The model under review builds one solid part; all positions refer to its coordinate system, in mm. A direction names the side the tool comes from. Give positions to 0.01 mm unless a question says otherwise; leave off trailing zeros. Order: outer loops, then holes, each group sorted by start corner. A loop starts at its lowest first (then second) coordinate and runs counter-clockwise, first axis right, second up.
```python
from build123d import *

# Parameters (mm, degrees)
F5_W      = 0.8128
F5_H      = 13.4112
F6_DEPTH  = 25.1968
F8_DEPTH  = 46.8002
F5_W_2    = 19.5072
F5_H_2    = 1.2
F5_W_3    = 5.1816
F5_H_3    = 11.592
F5_W_4    = 17.9008
F5_H_4    = 7.5376
F5_W_5    = 19.1008
F5_H_5    = 4.896
F5_W_6    = 1.2
F5_H_6    = 6.004279983
F9_DEPTH  = 19.4056
F5_W_7    = 4.6104
F5_H_7    = 5.8928
F5_W_8    = 6.1152
F5_H_8    = 4.712
F5_W_9    = 12.8016
F5_W_10   = 8.3888
F5_H_9    = 7.0104
F10_DEPTH = 17.9832
F11_DEPTH = 1.2192
F12_W     = 52.832
F12_H     = 38.2016
F12_W_2   = 1.0041694948
F12_H_2   = 6.004279983
F12_W_3   = 19.1008
F12_H_3   = 16.2133753487
F13_DEPTH = 0.913


with BuildPart() as f6:
    # F5 (on Top) → F6 (new body)
    with BuildSketch(Plane.XY):
        Polygon((0, 36.3344), (0, 0), (46.7992, 0), (46.7992, 1.2), (46.7992, 6.1976), (46.7992, 7.3976), (46.7992, 22.4344), (45.5992, 22.4344), (45.5992, 1.2), (1.2, 1.2), (1.2, 11.36), (1.2, 24.7712), (1.2, 35.1344), (45.5992, 35.1344), (45.5992, 31.864), (46.7992, 31.864), (46.7992, 36.3344), (15.2016, 36.3344), (14.0016, 36.3344), (1.2, 36.3344), align=None)
        with Locations((1.6064, 18.0656)):
            Rectangle(F5_W, F5_H)
    extrude(amount=F6_DEPTH)

    # F7 (on face) → F8 (cut, through all)
    with BuildSketch(Plane(origin=(0, 0, 0), x_dir=(0, -1, 0), z_dir=(-1, 0, 0))):
        Polygon((-35.1344, 25.1968), (0, 19.4056), (0, 25.1968), align=None)
    extrude(amount=-F8_DEPTH, mode=Mode.SUBTRACT)

    # F5 (on Top) → F9 (join)
    with BuildSketch(Plane.XY):
        Polygon((0, 103.7584), (0, 64.3568), (1.2, 64.3568), (1.2, 102.5584), (18.0656, 102.5584), (18.0656, 103.7584), align=None)
        with Locations((27.8192, 103.1584)):
            Rectangle(F5_W_2, F5_H_2)
        Polygon((120.5032, 103.7584), (37.5728, 103.7584), (37.5728, 102.5584), (54.032, 102.5584), (54.032, 64.3568), (55.232, 64.3568), (55.232, 102.5584), (99.0024, 102.5584), (99.0024, 93.8704553318), (100.2024, 93.8704553318), (101.2065694948, 93.8704553318), (101.2065694948, 87.8661753487), (100.2024, 87.8661753487), (99.0024, 87.8661753487), (99.0024, 70.4528), (100.2024, 70.4528), (100.2024, 86.6661753487), (102.4065694948, 86.6661753487), (119.3032, 86.6661753487), (119.3032, 70.4528), (120.5032, 70.4528), align=None)
        Polygon((100.2024, 95.0704553318), (100.2024, 102.5584), (119.3032, 102.5584), (119.3032, 87.8661753487), (102.4065694948, 87.8661753487), (102.4065694948, 95.0704553318), align=None, mode=Mode.SUBTRACT)
        Polygon((46.7992, 7.3976), (46.7992, 6.1976), (59.3152, 6.1976), (59.3152, -3.9624), (59.3152, -5.1624), (60.5152, -5.1624), (119.3032, -5.1624), (120.5032, -5.1624), (120.5032, 70.4528), (119.3032, 70.4528), (100.2024, 70.4528), (99.0024, 70.4528), (99.0024, 64.3568), (55.232, 64.3568), (54.032, 64.3568), (54.032, 63.1568), (66.6304, 63.1568), (66.6304, 36.3344), (67.8304, 36.3344), (67.8304, 63.1568), (119.3032, 63.1568), (119.3032, 49.5424), (100.2024, 49.5424), (100.2024, 36.3344), (101.4024, 36.3344), (101.4024, 39.6048), (119.3032, 39.6048), (119.3032, 21.6216), (107.2128, 21.6216), (107.2128, 20.4216), (119.3032, 20.4216), (119.3032, -3.9624), (92.4808, -3.9624), (92.4808, 20.4216), (91.2808, 20.4216), (91.2808, 8.8296), (86.0992, 8.8296), (86.0992, 20.4216), (84.8992, 20.4216), (84.8992, -3.9624), (60.5152, -3.9624), (60.5152, 20.4216), (59.3152, 20.4216), (59.3152, 7.3976), align=None)
        with Locations((88.69, 1.8336)):
            Rectangle(F5_W_3, F5_H_3, mode=Mode.SUBTRACT)
        with Locations((110.3528, 44.5736)):
            Rectangle(F5_W_4, F5_H_4, mode=Mode.SUBTRACT)
        with Locations((109.7528, 66.8048)):
            Rectangle(F5_W_5, F5_H_5, mode=Mode.SUBTRACT)
        with Locations((99.6024, 90.8683153403)):
            Rectangle(F5_W_6, F5_H_6)
    extrude(amount=F9_DEPTH)

    # F5 (on Top) → F10 (join)
    with BuildSketch(Plane.XY):
        Polygon((0, 64.3568), (0, 36.3344), (1.2, 36.3344), (1.2, 63.1568), (34.5248, 63.1568), (34.5248, 64.3568), (1.2, 64.3568), align=None)
        Polygon((59.3152, 21.6216), (59.3152, 20.4216), (60.5152, 20.4216), (84.8992, 20.4216), (86.0992, 20.4216), (91.2808, 20.4216), (92.4808, 20.4216), (107.2128, 20.4216), (107.2128, 21.6216), (107.2128, 28.7144), (101.4024, 28.7144), (101.4024, 36.3344), (100.2024, 36.3344), (67.8304, 36.3344), (66.6304, 36.3344), (59.3152, 36.3344), (59.3152, 29.2224), (91.4208, 29.2224), (91.4208, 35.1344), (100.2024, 35.1344), (100.2024, 21.6216), align=None)
        with Locations((103.7076, 24.568)):
            Rectangle(F5_W_7, F5_H_7, mode=Mode.SUBTRACT)
        with Locations((63.5728, 32.7784)):
            Rectangle(F5_W_8, F5_H_8, mode=Mode.SUBTRACT)
        with Locations((74.2312, 32.7784)):
            Rectangle(F5_W_9, F5_H_8, mode=Mode.SUBTRACT)
        with Locations((86.0264, 32.7784)):
            Rectangle(F5_W_10, F5_H_8, mode=Mode.SUBTRACT)
        with Locations((14.6016, 39.8396)):
            Rectangle(F5_W_6, F5_H_9)
    extrude(amount=F10_DEPTH)

    # F5 (on Top) → F11 (join)
    with BuildSketch(Plane.XY):
        Polygon((120.5032, 103.7584), (37.5728, 103.7584), (37.5728, 102.5584), (54.032, 102.5584), (54.032, 64.3568), (55.232, 64.3568), (55.232, 102.5584), (99.0024, 102.5584), (99.0024, 93.8704553318), (100.2024, 93.8704553318), (101.2065694948, 93.8704553318), (101.2065694948, 87.8661753487), (100.2024, 87.8661753487), (99.0024, 87.8661753487), (99.0024, 70.4528), (100.2024, 70.4528), (100.2024, 86.6661753487), (102.4065694948, 86.6661753487), (119.3032, 86.6661753487), (119.3032, 70.4528), (120.5032, 70.4528), align=None)
        Polygon((100.2024, 95.0704553318), (100.2024, 102.5584), (119.3032, 102.5584), (119.3032, 87.8661753487), (102.4065694948, 87.8661753487), (102.4065694948, 95.0704553318), align=None, mode=Mode.SUBTRACT)
        with Locations((27.8192, 103.1584)):
            Rectangle(F5_W_2, F5_H_2)
        Polygon((0, 103.7584), (0, 64.3568), (1.2, 64.3568), (1.2, 102.5584), (18.0656, 102.5584), (18.0656, 103.7584), align=None)
        with Locations((99.6024, 90.8683153403)):
            Rectangle(F5_W_6, F5_H_6)
    extrude(amount=-F11_DEPTH)

    # F12 (on face) → F13 (join)
    with BuildSketch(Plane(origin=(0, 0, -1.2192), x_dir=(1, 0, 0), z_dir=(0, 0, -1))):
        with Locations((27.616, -83.4576)):
            Rectangle(F12_W, F12_H)
        Polygon((99.0024, -64.3568), (55.232, -64.3568), (55.232, -102.5584), (99.0024, -102.5584), (99.0024, -70.4528), align=None)
        Polygon((1.2, -64.3568), (0, -64.3568), (0, -103.7584), (120.5032, -103.7584), (120.5032, -70.4528), (119.3032, -70.4528), (119.3032, -86.6661753487), (100.2024, -86.6661753487), (100.2024, -70.4528), (99.0024, -70.4528), (99.0024, -102.5584), (55.232, -102.5584), (55.232, -64.3568), (54.032, -64.3568), (54.032, -102.5584), (1.2, -102.5584), align=None)
        Polygon((119.3032, -102.5584), (100.2024, -102.5584), (100.2024, -95.0704553318), (102.4065694948, -95.0704553318), (102.4065694948, -87.8661753487), (119.3032, -87.8661753487), align=None, mode=Mode.SUBTRACT)
        with Locations((100.7044847474, -90.8683153403)):
            Rectangle(F12_W_2, F12_H_2, mode=Mode.SUBTRACT)
        with Locations((109.7528, -78.5594876744)):
            Rectangle(F12_W_3, F12_H_3)
        Polygon((100.2024, -95.0704553318), (100.2024, -102.5584), (119.3032, -102.5584), (119.3032, -87.8661753487), (102.4065694948, -87.8661753487), (102.4065694948, -95.0704553318), align=None)
    extrude(amount=F13_DEPTH)


solid = f6.part
```
Item 1: Take a section at B-B (y = 45.5). Give the boundary of the cut face in (x, z), and give its area (3 significant figures).
Values found:
outline: (0, 0) - (1.2, 0) - (1.2, 17.98) - (0, 17.98) - close; (66.63, 0) - (67.83, 0) - (67.83, 19.41) - (66.63, 19.41) - close; (100.2, 0) - (101.4, 0) - (101.4, 19.41) - (100.2, 19.41) - close; (119.3, 0) - (120.5, 0) - (120.5, 19.41) - (119.3, 19.41) - close
area: 91.4 mm2
Item 2: For faces 1 (the flat face through (53, 6.198, 10)), 2 (the flat face through (77, 64.357, 10)), 3 (the flat face through (45.599, 34, 12)), list the 3-axis set-ups (+Z, -Z, +X, -X, +Y, -Y) from which the entire face can be reached by the end or side of a thin tool; tool diameter is ignored.
Values found:
face 1: +Z, -Z, -Y
face 2: +Z
face 3: +Z, -Z
Item 3: Take a section at A-A (x = 110). Give the number of separate pieces and of enclosed holes in the cut face, and give its area (3 significant figures).
Values found:
separate pieces: 7
enclosed holes: 0
area: 220 mm2
Item 4: Take a section at C-C (x = 21). Give the boundary of the cut face in (y, z).
Values found:
outline: (0, 0) - (1.2, 0) - (1.2, 19.6) - (0, 19.41) - close; (35.13, 0) - (36.33, 0) - (36.33, 25.2) - (35.13, 25.2) - close; (63.16, 0) - (64.36, 0) - (64.36, 17.98) - (63.16, 17.98) - close; (64.36, -2.13) - (103.76, -2.13) - (103.76, 19.41) - (102.56, 19.41) - (102.56, -1.22) - (64.36, -1.22) - close
Item 5: Take a section at D-D (y = 60). Give the boundary of the cut face in (x, z).
Values found:
outline: (0, 0) - (1.2, 0) - (1.2, 17.98) - (0, 17.98) - close; (66.63, 0) - (67.83, 0) - (67.83, 19.41) - (66.63, 19.41) - close; (119.3, 0) - (120.5, 0) - (120.5, 19.41) - (119.3, 19.41) - close
Item 6: For line 1 (X direction, y = 11, z = 4); line 2 (Y direction, x = 38.5, z = 8.5); line 3 (X direction, y = 49.5, z = 14.75), list the stretches that pass through material, from the lowest coordinate up.
Values found:
line 1: x = 0 to 1.2, 45.6 to 46.8, 59.32 to 60.52, 84.9 to 86.1, 91.28 to 92.48, 119.3 to 120.5
line 2: y = 0 to 1.2, 35.13 to 36.33, 102.56 to 103.76
line 3: x = 0 to 1.2, 66.63 to 67.83, 100.2 to 120.5
Item 7: Clearance check with flat-ended pins moving along their axes: pin 1 Ø1 at (y, z) = (55, 21) entering from +X; pin 2 Ø1.3 at (x, y) = (15, 38.5) entering from +Z; pin 3 Ø5.5 at (y, z) = (-1.5, 13) entering from -X; pin 4 Ø10 at (x, y) = (64.5, 58) entering from -Z. State where each tip first meets the part, or that it passes through.
Values found:
pin 1: passes through
pin 2: stops at z = 17.98
pin 3: stops at x = 0
pin 4: stops at z = 0
